Part model, mm, in its own coordinate system. A direction names the side the tool comes from. Give positions to 0.01 mm unless a question says otherwise; leave off trailing zeros. Order: outer loops, then holes, each group sorted by start corner. A loop starts at its lowest first (then second) coordinate and runs counter-clockwise, first axis right, second up. Notation, with made-up numbers: M 81,48 L 137,48 A27 ccw 137,75 Z; hole C -8.5,57.5 d8. An arc over 180 degrees is marked long. Answer as a JSON object with one key per item and string values.
Autodesk Inventor part; units mm, degrees
ref_plane "YZ-Ebene" through (0, 0, 0) normal (1, 0, 0) x (0, 1, 0)
ref_plane "XZ-Ebene" through (0, 0, 0) normal (0, 1, 0) x (-1, 0, 0)
ref_plane "XY-Ebene" through (0, 0, 0) normal (0, 0, 1) x (1, 0, 0)
sketch "Skizze1" plane through (0, 0, 0) normal (0, 1, 0) x (-1, 0, 0)
  line L0 (-0.8169, 1.8861) -> (9.1831, 1.8861)
  line L1 (9.1831, 1.8861) -> (9.1831, -14.7439)
  line L2 (9.1831, -14.7439) -> (-0.8169, -14.7439)
  line L3 (-0.8169, -14.7439) -> (-0.8169, 1.8861)
  line L4 (-0.8169, 1.8861) -> (-10.2882, 21.743)
  line L5 (9.1831, 14.3218) -> (9.1831, 1.8861)
  line L6 (9.1831, 1.8861) -> (-2.1416, 25.6287)
  line L7 (-2.1416, 25.6287) -> (-10.2882, 21.743)
  point P0 (-5.5526, 11.8145)
  point P1 (9.1831, -3.6782)
  dimension "d23" = 154.5
  dimension "d24" = 10
  dimension "d25" = 22
  dimension "d26" = 16.63
  dimension "d27" = 9.9284
extrude "Extrusion3" add sketch "Skizze1" along normal blind 28
sketch "Skizze4" plane through (0.8169, 0, 1.8861) normal (0.9026, 0, -0.4305) x (-0.4305, 0, -0.9026)
  circle A0 centre (-4.65, 24.16) radius 2.5
  circle A1 centre (-4.65, 3.84) radius 2.5
  circle A2 centre (-17.35, 3.84) radius 2.5
  circle A3 centre (-17.35, 24.16) radius 2.5
  line L0 (-22, 28) -> (0, 28)
  line L1 (-22, 0) -> (-22, 28)
  line L2 (0, 0) -> (0, 28)
  circle A4 centre (-4.65, 24.16) radius 1.5
  circle A5 centre (-4.65, 3.84) radius 1.5
  circle A6 centre (-17.35, 3.84) radius 1.5
  circle A7 centre (-17.35, 24.16) radius 1.5
  point P0 (2.0541, 0)
  dimension "d35" = 5
  dimension "d36" = 5
  dimension "d37" = 5
  dimension "d38" = 5
  dimension "d39" = 20.32
  dimension "d40" = 20.32
  dimension "d41" = 12.7
  dimension "d42" = 12.7
  dimension "d43" = 3.84
  dimension "d45" = 4.65
  dimension "d46" = 4.65
  dimension "d47" = 3.84
  dimension "d48" = 3
  dimension "d49" = 3
  dimension "d50" = 3
  dimension "d51" = 3
extrude "Extrusion4" add sketch "Skizze4" along normal blind 5
extrude "Extrusion5" cut sketch "Skizze4" against normal blind 10 contours A4 | A5 | A6 | A7
sketch "Skizze6" plane through (-9.1831, 0, -14.7439) normal (-1, 0, 0) x (0, 0, 1)
  line L0 (0, 0) -> (16.63, 0)
  line L1 (0, 28) -> (16.63, 28)
  line L2 (0, 0) -> (3, 0)
  line L3 (3, 0) -> (3, 28)
  line L4 (3, 28) -> (0, 28)
  line L5 (0, 28) -> (0, 0)
  point P0 (14.7439, 0)
  point P1 (36.0154, 0)
  point P2 (36.0154, 28)
  point P3 (3, 0)
  dimension "d56" = 3
extrude "Extrusion6" add sketch "Skizze6" along normal blind 10
sketch "Skizze7" plane through (0.8169, 0, 1.8861) normal (1, 0, 0) x (0, 0, -1)
  line L0 (16.63, 0) -> (16.63, 28)
  line L1 (0, 0) -> (16.63, 0)
  line L2 (16.63, 28) -> (13.63, 28)
  line L3 (13.63, 28) -> (13.63, 0)
  line L4 (13.63, 0) -> (16.63, 0)
  line L5 (16.63, 0) -> (16.63, 28)
  point P0 (1.8861, 0)
  dimension "d59" = 3
extrude "Extrusion7" add sketch "Skizze7" along normal blind 10
sketch "Skizze8" plane through (0, 0, 0) normal (0, -1, 0) x (1, 0, 0)
  line L0 (0.8169, -11.7439) -> (10.8169, -11.7439)
  line L1 (10.8169, -11.7439) -> (0.8148, -1.7417)
  line L2 (10.8169, -11.7439) -> (24.9621, -11.7439) construction
  line L3 (-9.1831, -11.7439) -> (-19.1831, -11.7439)
  line L4 (-19.1831, -11.7439) -> (-9.1831, -1.7417)
  line L5 (-9.1831, -11.7439) -> (-9.1831, 1.8861)
  line L6 (10.8169, -14.7439) -> (10.8169, -11.7439)
  line L7 (10.8169, -11.7439) -> (-19.1831, -11.7439)
  line L8 (-9.1831, -1.7417) -> (0.8148, -1.7417)
  point P0 (0, 0)
  point P1 (-9.1831, 3.2715)
  point P2 (-9.1831, -11.7439)
  dimension "d62" = 135
extrude "Extrusion8" add sketch "Skizze8" against normal blind 3
sketch "Skizze9" plane through (0, 28, 0) normal (0, 1, 0) x (1, 0, 0)
  line L0 (-9.1831, 11.7439) -> (-19.1831, 11.7439)
  line L1 (-19.1831, 11.7439) -> (-9.1831, 1.7417)
  line L2 (-9.1831, 1.7417) -> (0.8169, 1.7417)
  line L3 (0.8169, -1.8861) -> (0.8169, 11.7439)
  line L4 (10.8169, 14.7439) -> (10.8169, 11.7439)
  line L5 (10.8169, 11.7439) -> (0.8169, 1.7417)
  line L6 (-19.1831, 11.7439) -> (10.8169, 11.7439)
  point P0 (0, 0)
  point P1 (-9.1831, 11.7439)
extrude "Extrusion9" add sketch "Skizze9" against normal blind 3
sketch "Skizze10" plane through (-19.1831, 0, -14.7439) normal (0, 0, -1) x (-1, 0, 0)
  circle A0 centre (-5, 14) radius 2
  circle A1 centre (-25, 14) radius 2
  line L0 (0, 28) -> (0, 0)
  line L1 (-30, 0) -> (-30, 28)
  line L2 (0, 0) -> (-30, 0)
  point P0 (-19.1831, 0)
  dimension "d67" = 4
  dimension "d68" = 4
  dimension "d69" = 5
  dimension "d70" = 5
  dimension "d71" = 14
  dimension "d72" = 14
extrude "Extrusion10" cut sketch "Skizze10" against normal blind 50
sketch "Skizze11" plane through (0, 28, 0) normal (0, 1, 0) x (1, 0, 0)
  line L0 (10.8169, 14.7439) -> (10.8169, 11.7439)
  line L1 (-19.1831, 14.7439) -> (10.8169, 14.7439)
  line L2 (-19.1831, 11.7439) -> (-19.1831, 14.7439)
  line L3 (-19.1831, 11.7439) -> (-9.1831, 1.7417)
  line L4 (-9.1831, 1.7417) -> (-9.1831, -1.8861)
  line L5 (-9.1831, -1.8861) -> (2.1416, -25.6287)
  line L6 (2.1416, -25.6287) -> (10.2882, -21.743)
  line L7 (10.2882, -21.743) -> (0.8169, -1.8861)
  line L8 (0.8169, -1.8861) -> (0.8169, 1.7417)
  line L9 (0.8169, 1.7417) -> (10.8169, 11.7439)
  line L10 (-9.1831, 1.7417) -> (-9.1831, -1.8861)
  line L11 (-9.1831, -1.8861) -> (2.1416, -25.6287)
  line L12 (-9.1831, 1.7417) -> (-9.1831, -1.6598)
  line L13 (-9.0856, -2.0903) -> (1.7111, -24.7261)
  line L14 (2.1416, -25.6287) -> (10.2882, -21.743)
  line L15 (3.0442, -25.1982) -> (9.3856, -22.1735)
  line L16 (0.8169, -1.8861) -> (0.8169, 1.7417)
  line L17 (0.8169, 19.7417) -> (0.8169, -1.6598)
  line L18 (0.9144, -2.0903) -> (9.8577, -20.8404)
  arc A0 (-9.1831, -1.6598) -> (-9.0856, -2.0903) centre (-8.1831, -1.6598) ccw
  arc A1 (1.7111, -24.7261) -> (3.0442, -25.1982) centre (2.6137, -24.2956) ccw
  arc A2 (9.3856, -22.1735) -> (9.8577, -20.8404) centre (8.9551, -21.2709) ccw
  arc A3 (0.8169, -1.6598) -> (0.9144, -2.0903) centre (1.8169, -1.6598) ccw
  point P0 (0, 0)
  point P1 (9.3856, -22.1735)
  point P2 (3.0442, -25.1982)
  point P3 (1.7111, -24.7261)
  point P4 (-9.1831, -1.6598)
  point P5 (0.9144, -2.0903)
  point P6 (0.8169, -1.6598)
  dimension "d75" = 1
  dimension "d76" = 1
extrude "Extrusion11" cut sketch "Skizze11" against normal blind 30 contours L7 L6 A2 | A0 L5 L4 | L6 L5 A1
extrude "Extrusion12" add sketch "Skizze11" against normal blind 28 contours A3 L7 L8
chamfer "Fase3" distance 0.6 angle 45 1 edges at (9.3626, 24.16, 19.8024)
chamfer "Fase4" distance 0.6 angle 45 1 edges at (9.3626, 3.84, 19.8024)
chamfer "Fase5" distance 0.6 angle 45 2 edges at (3.8951, 24.16, 8.3396) (3.8951, 3.84, 8.3396)
properties part number "ir_camera_mount"
1. Cut at D-D on z = 12. Give the cut face in (x, y).
Worked answers:
{"outline": "M -4.36,0 L 5.64,0 L 5.64,12.01 A2 cw 5.64,15.99 L 5.64,28 L -4.36,28 Z"}
2. Two-plate mould, pull along Z, no slides. Class faces 1 (the flat face through (6.63, 3.32, 2.46)), 2 (the flat face through (-4, 14, -14.744)), 3 (the flat face through (-19.183, 14, -13)): +Z half, -Z half, draft (parallel to the pull), parting line (faces both ways), or undercut.
Worked answers:
{"face 1": "undercut", "face 2": "-Z half", "face 3": "draft"}
3. Probe line 1 along Z through (x, y) = (8, 25.25); line 2 along X through (y, z) = (11, 1.5); line 3 along Z through (x, y) = (4, 23.75). List the from-to ranges inside material, lowest first.
Worked answers:
{"line 1": "z = -14.74 to -8.93, 5.33 to 6.1, 15.19 to 16.54, 18.82 to 22.83", "line 2": "x = -9.18 to 0.82", "line 3": "z = -14.74 to -11.74, 2.79 to 3.92, 7.12 to 17.99, 21.19 to 24.74"}
4. Pin check, flat tips, straight feed: P1, Ø6, axis at x = -8, z = 12, coming from the +Y side (3 decimals); P2, Ø1.5, axis at y = 9.5, z = -13.5, coming from the +X side; P3, Ø1.5, axis at x = 4.5, z = 6, coming from the +Y side; P4, Ø4, axis at y = 10, z = -3.5, coming from the +X side. Stop position of each tip, or through.
Worked answers:
{"P1": "passes through", "P2": "stops at x = 10.82", "P3": "stops at y = 26.66", "P4": "stops at x = 0.82"}
5. Which spindle directions (+Z, -Z, +X, -X, +Y, -Y) get a long thin tool onto all of the face, cutting with end or side? Do faces 4 (the flat face through (0.817, 14, -5)), 5 (the flat face through (5.887, 26.521, -6.813)), 6 (the flat face through (-16.34, 13.85, -11.744)). Say none if no direction does.
Worked answers:
{"face 4": "+X", "face 5": "+X, +Y, -Y", "face 6": "+Z, -X"}
6. Cut at A-A on y = 14. Give the cut face in (x, z).
Worked answers:
{"outline": "M -19.18,-14.74 L -16.18,-14.74 L -16.18,-11.74 L -19.18,-11.74 Z; M -12.18,-14.74 L 3.82,-14.74 L 3.82,-11.74 L 0.82,-11.74 L 0.82,1.66 A1 cw 0.91,2.09 L 3.82,8.18 L 3.82,24.83 L 3.04,25.2 A1 ccw 1.71,24.73 L -9.09,2.09 A1 ccw -9.18,1.66 L -9.18,-11.74 L -12.18,-11.74 Z; M 7.82,-14.74 L 10.82,-14.74 L 10.82,-11.74 L 7.82,-11.74 Z; M 7.82,16.56 L 9.86,20.84 A1 ccw 9.39,22.17 L 7.82,22.92 Z"}
7. Cut at C-C on z = -4. Give the cut face in (x, y).
Worked answers:
{"outline": "M -11.44,0 L 3.07,0 L 3.07,3 L 0.82,3 L 0.82,25 L 3.07,25 L 3.07,28 L -11.44,28 L -11.44,25 L -9.18,25 L -9.18,3 L -11.44,3 Z"}
8. Cut at B-B on x = -14. Give the cut face in (y, z), plus the area to 3 significant figures.
Worked answers:
{"outline": "M 0,-14.74 L 12.01,-14.74 L 12.01,-11.74 L 3,-11.74 L 3,-6.56 L 0,-6.56 Z; M 15.99,-14.74 L 28,-14.74 L 28,-6.56 L 25,-6.56 L 25,-11.74 L 15.99,-11.74 Z", "area": "103 mm^2"}
